from build123d import *

# Parameters (mm, degrees)
F0_W     = 80
F0_H     = 45
F1_DEPTH = 25
F2_R     = 12
F3_DEPTH = 2
F4_R     = 3.5
F5_DEPTH = 6
F6_R     = 20


with BuildPart() as f1:
    # F0 (on Top) → F1 (new body)
    with BuildSketch(Plane.XY):
        Rectangle(F0_W, F0_H)
    extrude(amount=F1_DEPTH)

    # F2 (on face) → F3 (cut)
    with BuildSketch(Plane.XY.offset(25)):
        with Locations((-20, 0)):
            Circle(F2_R)
        with Locations((20, 0)):
            Circle(F2_R)
    extrude(amount=-F3_DEPTH, mode=Mode.SUBTRACT)

    # F4 (on face) → F5 (cut)
    with BuildSketch(Plane.XY.offset(23)):
        with Locations((-20, 0)):
            Circle(F4_R)
        with Locations((20, 0)):
            Circle(F4_R)
    extrude(amount=-F5_DEPTH, mode=Mode.SUBTRACT)

    # F6
    f6_edges = [f1.edges().sort_by_distance(p)[0] for p in [
        (-40, -22.5, 12.5),
        (-40, 22.5, 12.5),
        (40, -22.5, 12.5),
        (40, 22.5, 12.5),
    ]]
    fillet(f6_edges, radius=F6_R)


solid = f1.part
Geometry check sheet. Reference: the model listing, model coordinates, mm. A direction names the side the tool comes from. Round coordinates to 2 decimals unless told otherwise and drop trailing zeros. Loops run counter-clockwise (first coordinate to the right, second up) from the corner with the lowest first, then second, coordinate; pieces in that order, holes last. Notation, with made-up numbers: (-22, 4.25) - (-3, 4.25) arc R16 ccw to (-3, 27.25) - close; hole circle Ø3 at (-40, -6.75). An arc over 180 degrees is marked (long way). Answer as CSV lines item,"result".
(1) Release check for a two-part mould opening along Y. For faces 1 (the face through (-17.5, 2.8, 23)), 2 (the face through (40, 0, 12)), 3 (the face through (-8.554, 3.604, 24.014)), 4 (the face through (-34.297, 16.486, 12.675)) record: released by +Y, released by -Y, zero draft, split by the parting line, or undercut.
Output values:
face 1,"undercut"
face 2,"zero draft"
face 3,"undercut"
face 4,"released by +Y"
(2) Material ranges on line 1 along Y through (x, z) = (-20, 24.65); line 2 along Z through (x, y) = (11, 3); line 3 along X through (y, z) = (-7, 20.5), recorded low to high.
Output values:
line 1,"y = -22.5 to -12, 12 to 22.5"
line 2,"z = 0 to 23"
line 3,"x = -39.49 to 39.49"
(3) Cross-section at A-A, the plane z = 9.25. Enter the section's corners in (x, y), and give its area (3 significant figures).
Output values:
outline,"(-40, -2.5) arc R20 ccw to (-20, -22.5) - (20, -22.5) arc R20 ccw to (40, -2.5) - (40, 2.5) arc R20 ccw to (20, 22.5) - (-20, 22.5) arc R20 ccw to (-40, 2.5) - close"
area,"3,260 mm²"
(4) Depth check by flat-ended pin: pin 1 Ø1 at (y, z) = (17.5, 22) entering from +X (3 decimals); pin 2 Ø5.5 at (x, y) = (21.5, 0) entering from +Z; pin 3 Ø6 at (x, z) = (27.5, 16.5) entering from +Y. Enter the tip coordinate at first touch or a pass-through.
Output values:
pin 1,"stops at x = 33.775"
pin 2,"stops at z = 23"
pin 3,"stops at y = 21.99"
(5) Set-up check for faces 5 (the face through (-16.66, 1.05, 20.04)), 6 (the face through (0, 22.5, 12)): record each of +Z, -Z, +X, -X, +Y, -Y from which the full face is reachable in a straight line by a thin tool's end or side.
Output values:
face 5,"+Z"
face 6,"+Z, -Z, +X, -X, +Y"
(6) Cross-section at D-D, the plane x = -19. Enter the section's corners in (y, z).
Output values:
outline,"(-22.5, 0) - (22.5, 0) - (22.5, 25) - (11.96, 25) - (11.96, 23) - (3.35, 23) - (3.35, 17) - (-3.35, 17) - (-3.35, 23) - (-11.96, 23) - (-11.96, 25) - (-22.5, 25) - close"
(7) Cross-section at B-B, the plane y = 0. Enter the section's corners in (x, z).
Output values:
outline,"(-40, 0) - (40, 0) - (40, 25) - (32, 25) - (32, 23) - (23.5, 23) - (23.5, 17) - (16.5, 17) - (16.5, 23) - (8, 23) - (8, 25) - (-8, 25) - (-8, 23) - (-16.5, 23) - (-16.5, 17) - (-23.5, 17) - (-23.5, 23) - (-32, 23) - (-32, 25) - (-40, 25) - close"
(8) Cross-section at C-C, the plane z = 19. Enter the section's corners in (x, y), and give its area (3 significant figures).
Output values:
outline,"(-40, -2.5) arc R20 ccw to (-20, -22.5) - (20, -22.5) arc R20 ccw to (40, -2.5) - (40, 2.5) arc R20 ccw to (20, 22.5) - (-20, 22.5) arc R20 ccw to (-40, 2.5) - close; hole circle Ø7 at (-20, 0); hole circle Ø7 at (20, 0)"
area,"3,180 mm²"
